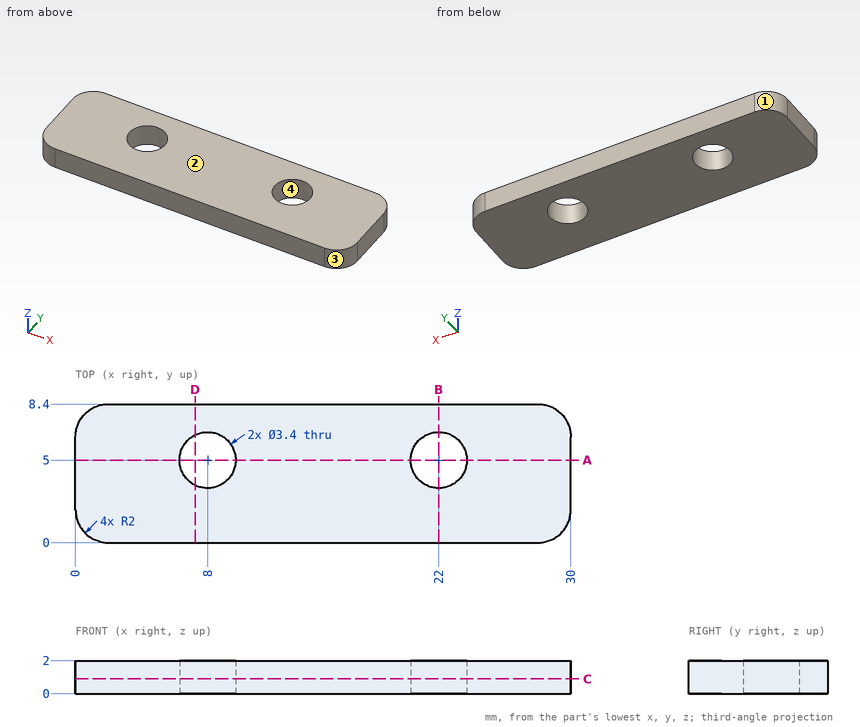
Geometry: see drawing. Coordinates: mm, zero at the bounding-box minimum. Give positions to 0.01 mm unless a question says otherwise; leave off trailing zeros. Loops run counter-clockwise (first coordinate to the right, second up) from the corner with the lowest first, then second, coordinate; pieces in that order, holes last. Notation, with made-up numbers: (-17.75, 40) - (23.25, 40) arc R20 ccw to (23.25, 74) - close; hole circle Ø11 at (77, 75). An arc over 180 degrees is marked (long way). Answer as CSV lines item,"result". Start each with the question number.
1. Section A-A, the plane y = 5. Return loops of the section in (x, z), plus the area to 3 significant figures.
2. Section D-D, the plane x = 7.25. Return loops of the section in (y, z), plus the area to 3 significant figures.
3. Section B-B, the plane x = 22. Return loops of the section in (y, z), plus the area to 3 significant figures.
4. Section C-C, the plane z = 0.9. Return loops of the section in (x, y), plus the area to 3 significant figures.
5. Ray query, L1, parallel to Y at x = 22, z = 1; L2, parallel to X at y = 5.25, z = 0.35; L3, parallel to X at y = 4.5, z = 0.25. Return the intervals inside material, ascending.
6. Draft query along X for the marked faces 1, 2, 3 and 4. Return one class per face: released by +X, released by -X, zero draft, split by the parting line, or undercut.
Answers:
1,outline,"(0, 0) - (6.3, 0) - (6.3, 2) - (0, 2) - close; (9.7, 0) - (20.3, 0) - (20.3, 2) - (9.7, 2) - close; (23.7, 0) - (30, 0) - (30, 2) - (23.7, 2) - close"
1,area,"46.4 mm2"
2,outline,"(0, 0) - (3.47, 0) - (3.47, 2) - (0, 2) - close; (6.53, 0) - (8.4, 0) - (8.4, 2) - (6.53, 2) - close"
2,area,"10.7 mm2"
3,outline,"(0, 0) - (3.3, 0) - (3.3, 2) - (0, 2) - close; (6.7, 0) - (8.4, 0) - (8.4, 2) - (6.7, 2) - close"
3,area,"10.0 mm2"
4,outline,"(0, 2) arc R2 ccw to (2, 0) - (28, 0) arc R2 ccw to (30, 2) - (30, 6.4) arc R2 ccw to (28, 8.4) - (2, 8.4) arc R2 ccw to (0, 6.4) - close; hole circle Ø3.4 at (8, 5); hole circle Ø3.4 at (22, 5)"
4,area,"230 mm2"
5,L1,"y = 0 to 3.3, 6.7 to 8.4"
5,L2,"x = 0 to 6.32, 9.68 to 20.32, 23.68 to 30"
5,L3,"x = 0 to 6.38, 9.62 to 20.38, 23.62 to 30"
6,face 1,"released by -X"
6,face 2,"zero draft"
6,face 3,"released by +X"
6,face 4,"undercut"
